Here's how the part is built. I have some questions about the finished solid (model axes, mm). Face numbers are marked on the shaded views. A direction names the side the tool comes from. Round coordinates to 2 decimals unless told otherwise and drop trailing zeros. Write each loop counter-clockwise with the first axis right and the second up, starting at its lowest first coordinate (ties: lowest second). Pieces come first, ordered by that corner, then holes. Notation, with made-up numbers: (75, 50.25) -> (98, 50.25) arc R13 cw to (98, 69.25) -> close; hole circle Ø2 at (-35.5, 24). An arc over 180 degrees is marked (long way). Answer as CSV lines item,"result".
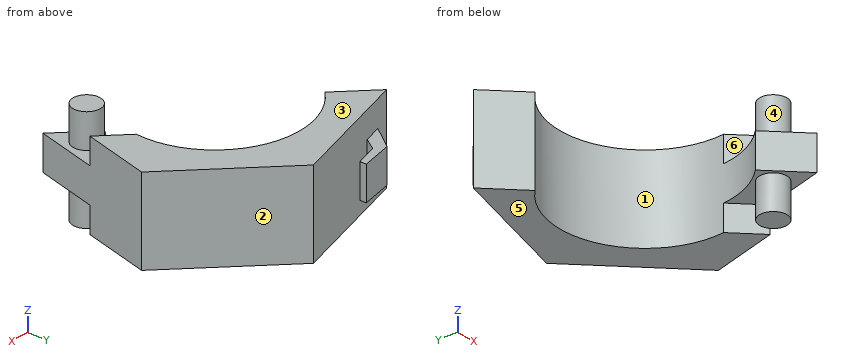
from build123d import *

# Parameters (mm, degrees)
BOSS_EXTRUDE1_DEPTH = 25.4
CUT_EXTRUDE1_DEPTH  = 7.62
SKETCH3_R           = 4
BOSS_EXTRUDE2_DEPTH = 10
BOSS_EXTRUDE3_DEPTH = 5


with BuildPart() as part:
    # Sketch1 → Boss-Extrude1 (new body)
    with BuildSketch(Plane.XY):
        with BuildLine():
            Line((9.541145468, 37.814898429), (-27.978089947, 27.17032357))
            Line((-27.978089947, 27.17032357), (-17.934673043, 17.416874084))
            ThreePointArc((-17.934673043, 17.416874084), (17.416874084, 17.934673043), (17.934673043, -17.416874084))
            Line((17.934673043, -17.416874084), (27.978089947, -27.17032357))
            Line((27.978089947, -27.17032357), (37.519235415, 10.644574858))
            Line((37.519235415, 10.644574858), (9.541145468, 37.814898429))
        make_face()
    extrude(amount=BOSS_EXTRUDE1_DEPTH)

    # Sketch2 → Cut-Extrude1 (cut)
    with BuildSketch(Plane.XY.offset(25.4)):
        Polygon((21.419411921, 1.52926165), (45.089583043, -21.457518704), (5.352657375, -38.695482799), align=None)
    cut_extrude1 = extrude(amount=-CUT_EXTRUDE1_DEPTH, mode=Mode.SUBTRACT)

    # Sketch3 → Boss-Extrude2 (add)
    with BuildSketch(Plane.XY.offset(17.78)):
        with Locations((24.578895169, -17.023104028)):
            Circle(SKETCH3_R)
    boss_extrude2 = extrude(amount=BOSS_EXTRUDE2_DEPTH)

    # Mirror1: Cut-Extrude1, Boss-Extrude2 across plane
    add(cut_extrude1.mirror(Plane(origin=(0, 0, 12.7), x_dir=(1, 0, 0), z_dir=(0, 0, -1))), mode=Mode.SUBTRACT)
    add(boss_extrude2.mirror(Plane(origin=(0, 0, 12.7), x_dir=(1, 0, 0), z_dir=(0, 0, -1))))

    # Sketch4 → Boss-Extrude3 (add, symmetric)
    with BuildSketch(Plane(origin=(0, 0, 12.7), x_dir=(-1, 0, 0), z_dir=(0, 0, -1))):
        Polygon((23.45113357, 28.454665469), (18.442827964, 35.547681457), (9.125788769, 37.439046087), (9.125788769, 35.547681457), (15.649252306, 33.696910907), (17.983802714, 30.005800825), align=None)
    extrude(amount=BOSS_EXTRUDE3_DEPTH, both=True)


solid = part.part
Item 1: If we mould it in two halves opening along X, with no side actions, what happens to the marked faces 1, 2 and 3? For each: pulls with the +X half, pulls with the -X half, needs draft (parallel to the pull), parting line crosses it, or undercut.
Results found:
face 1,"undercut"
face 2,"pulls with the +X half"
face 3,"needs draft"
Item 2: For the marked faces 4, 5 and 6, which set-ups out of +Z, -Z, +X, -X, +Y, -Y let a thin tool reach every point of the face, with its end or its side?
Results found:
face 4,"+Z"
face 5,"-Z, +X, -X, +Y"
face 6,"+Z, -X"
Item 3: Suppose I cut it at B-B, the plane x = -11. List the corners of the cut face in (y, z) for me.
Results found:
outline,"(22.45, 0) -> (31.99, 0) -> (31.99, 25.4) -> (22.45, 25.4) -> close; (35.02, 7.7) -> (37.06, 7.7) -> (37.06, 17.7) -> (35.02, 17.7) -> close"
Item 4: Will these pins go through, and if not, where does the flat tip stop? pin 1 (4.5 mm diameter, centred on x = -14.5, y = 33.5, fed in from -Z); pin 2 (1.5 mm diameter, centred on x = 25, y = 15, fed in from +Z); pin 3 (8 mm diameter, centred on y = 24, z = 22, fed in from +X).
Results found:
pin 1,"stops at z = 7.7"
pin 2,"stops at z = 25.4"
pin 3,"stops at x = 27.89"
Item 5: Suppose I cut it at D-D, the plane y = -8. List the corners of the cut face in (x, z) for me, then the cut area to 3 significant figures.
Results found:
outline,"(23.69, 7.62) -> (31.23, 7.62) -> (31.23, 0) -> (32.81, 0) -> (32.81, 25.4) -> (31.23, 25.4) -> (31.23, 17.78) -> (23.69, 17.78) -> close"
area,"117 mm²"
Item 6: Suppose I cut it at C-C, the plane y = 23. List the corners of the cut face in (x, z) for me, then the cut area to 3 significant figures.
Results found:
outline,"(-23.68, 0) -> (-9.8, 0) -> (-9.8, 25.4) -> (-23.68, 25.4) -> close; (9.8, 0) -> (24.8, 0) -> (24.8, 25.4) -> (9.8, 25.4) -> close"
area,"734 mm²"
Item 7: I need wall thicknesses on L1, parallel to Z at x = 29.5, y = -8; L2, parallel to Z at x = 25, y = 13.5; L3, parallel to X at y = 22, z = 1.5. Which ranges of each line are inside material? Lowest first, please.
Results found:
L1,"z = 7.62 to 17.78"
L2,"z = 0 to 25.4"
L3,"x = -22.65 to -11.87, 11.87 to 25.83"
Item 8: Suppose I cut it at A-A, the plane z = 22. List the corners of the cut face in (x, y) for me.
Results found:
outline,"(-27.98, 27.17) -> (-17.93, 17.42) arc R25 cw to (24.93, -1.88) -> (32.5, -9.23) -> (37.52, 10.64) -> (9.54, 37.81) -> close; circle Ø8 at (24.58, -17.02)"
